Here's how the part is built. I have some questions about the finished solid (model axes, mm). Face numbers are marked on the shaded views. A direction names the side the tool comes from. Give positions to 0.01 mm unless a question says otherwise; leave off trailing zeros. Order: outer loops, then holes, each group sorted by start corner. A loop starts at its lowest first (then second) coordinate and runs counter-clockwise, first axis right, second up. Notation, with made-up numbers: (26, 63) -> (57, 63) arc R21 ccw to (57, 99) -> close; hole circle Ø3 at (68, 31.25). An arc over 180 degrees is marked (long way). Write each question's results on one line, items separated by ' | '. Start each with the question number.
Q1. Thinking about a two-plate mould opening in Z: for the marked faces 1, 2, 3 and 4, which applies, pulls with the +Z half, pulls with the -Z half, needs draft (parallel to the pull), parting line crosses it, or undercut?
Q2. Imagine slicing it at A-A, the plane z = 32.5. Please give me the cut outline in (x, y).
Q3. For the marked faces 5 and 6, which set-ups out of +Z, -Z, +X, -X, +Y, -Y let a thin tool reach every point of the face, with its end or its side?
Q4. I need wall thicknesses on line 1 along Z through (x, y) = (-45.75, 0.5); line 2 along X through (y, z) = (1.3, 32.5); line 3 along Z through (x, y) = (-55.5, 1.25). Which ranges of each line are inside material? Lowest first, please. Write a range as [from, to].
Q5. Imagine slicing it at B-B, the plane y = 3.75. Please give me the cut outline in (x, z).
Q6. Imagine slicing it at D-D, the plane z = 7.5. Please give me the cut outline in (x, y).
Q7. Imagine slicing it at C-C, the plane x = -46. Please give me the cut outline in (y, z).
Q8. I'm going to push flat-ended pins straight in: pin 1 (2 mm diameter, centred on y = 6, z = 17, fed in from +X); pin 2 (1.5 mm diameter, centred on x = -49, y = 5.5, fed in from +Z); pin 3 (7 mm diameter, centred on x = -54.75, z = 32.5, fed in from -Y); pin 4 (3.5 mm diameter, centred on x = -44.23, y = 3.75, fed in from -Z). Where does each tip first touch, or does it pass through?
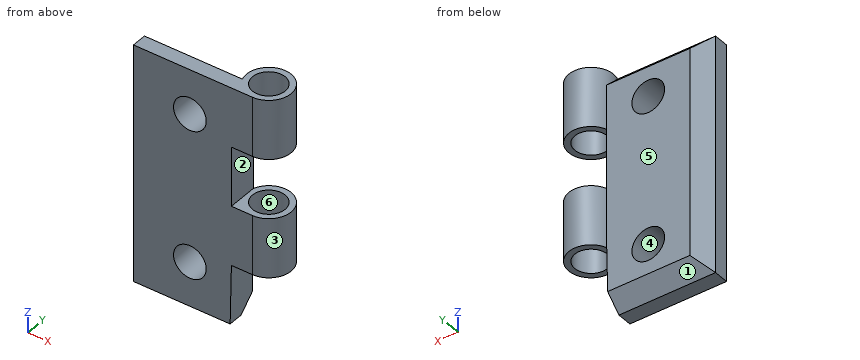
```python
from build123d import *

# Parameters (mm, degrees)
IZIM1_R                     = 2.75
Y_KSEKLIK_EKSTR_ZYON1_DEPTH = 40
PAH3_SIZE                   = 2.5
IZIM2_R                     = 2.75
IZIM2_W                     = 7.285533906
IZIM2_H                     = 10
KES_EKSTR_ZYON1_DEPTH       = 40
KES_EKSTR_ZYON2_DEPTH       = 88


with BuildPart() as part:
    # Çizim1 → Yükseklik-Ekstrüzyon1 (new body)
    with BuildSketch(Plane.XY):
        with BuildLine():
            Line((-64.233873571, 5), (-64.233873571, 0))
            Line((-64.233873571, 0), (-44.233873571, 0))
            ThreePointArc((-44.233873571, 0), (-41.172011393, 5.915063509), (-47.769407477, 5))
            Line((-47.769407477, 5), (-64.233873571, 5))
        make_face()
        with Locations((-44.233873571, 3.75)):
            Circle(IZIM1_R, mode=Mode.SUBTRACT)
    extrude(amount=Y_KSEKLIK_EKSTR_ZYON1_DEPTH)

    # Pah3
    pah3_edges = [part.edges().sort_by_distance(p)[0] for p in [
        (-56.001640524, 5, 40),
        (-56.001640524, 5, 0),
        (-64.233873571, 5, 20),
    ]]
    chamfer(pah3_edges, length=PAH3_SIZE)

    # Çizim2 → Kes-Ekstrüzyon1 (cut)
    with BuildSketch(Plane(origin=(0, 0, 0), x_dir=(1, 0, 0), z_dir=(0, 1, 0))):
        with Locations(Location((-54.751640524, -32.5, 0), (0, 0, 90))):
            Circle(IZIM2_R)
        with Locations(Location((-54.751640524, -7.5, 0), (0, 0, 90))):
            Circle(IZIM2_R)
        with Locations((-44.126640524, -25)):
            Rectangle(IZIM2_W, IZIM2_H)
        Polygon((-40.483873571, 0), (-47.983873571, 0), (-47.769407477, -10), (-40.483873571, -10), align=None)
    extrude(amount=KES_EKSTR_ZYON1_DEPTH, mode=Mode.SUBTRACT)

    # Çizim3 → Kes-Ekstrüzyon2 (cut)
    with BuildSketch(Plane(origin=(0, 0, 0), x_dir=(0, 0, -1), z_dir=(1, 0, 0))):
        Polygon((-0.875256962, 3.375256962), (-1.784369295, 4.284369295), (0.59171966, 4.284369295), (0.36885853, 3.16350742), align=None)
    extrude(amount=-KES_EKSTR_ZYON2_DEPTH, mode=Mode.SUBTRACT)


solid = part.part
```
Geometry check:
1) face 1: pulls with the -Z half | face 2: undercut | face 3: needs draft | face 4: undercut
2) outline: (-64.23, 0) -> (-57.5, 0) -> (-57.5, 5) -> (-61.73, 5) -> (-64.23, 2.5) -> close; (-52, 0) -> (-44.23, 0) arc R3.75 ccw (long way) to (-47.77, 5) -> (-52, 5) -> close; hole circle Ø5.5 at (-44.23, 3.75)
3) face 5: +Z, -Z, -X, +Y | face 6: +Z, -Z
4) line 1: [10, 20], [30, 40] | line 2: [-64.23, -57.5], [-52, -45.48], [-42.98, -41.39] | line 3: [0, 4.85], [10.15, 29.85], [35.15, 40]
5) outline: (-62.98, 1.25) -> (-47.96, 1.25) -> (-47.77, 10) -> (-46.98, 10) -> (-46.98, 20) -> (-47.77, 20) -> (-47.77, 30) -> (-46.98, 30) -> (-46.98, 40) -> (-47.98, 40) -> (-47.98, 38.75) -> (-62.98, 38.75) -> close; (-41.48, 10) -> (-40.48, 10) -> (-40.48, 20) -> (-41.48, 20) -> close; (-41.48, 30) -> (-40.48, 30) -> (-40.48, 40) -> (-41.48, 40) -> close; hole circle Ø5.5 at (-54.75, 7.5); hole circle Ø5.5 at (-54.75, 32.5)
6) outline: (-64.23, 0) -> (-57.5, 0) -> (-57.5, 5) -> (-61.73, 5) -> (-64.23, 2.5) -> close; (-52, 0) -> (-47.82, 0) -> (-47.82, 5) -> (-52, 5) -> close
7) outline: (0, 10) -> (1.64, 10) -> (1.64, 20) -> (0, 20) -> close; (0, 30) -> (1.64, 30) -> (1.64, 40) -> (0, 40) -> close; (5.86, 10) -> (7.06, 10) -> (7.06, 20) -> (5.86, 20) -> close; (5.86, 30) -> (7.06, 30) -> (7.06, 40) -> (5.86, 40) -> close
8) pin 1: x = -40.7 | pin 2: z = 37.75 | pin 3: y = 0 | pin 4: through
